Read the model definition and answer for the solid it produces. Units are mm, in the model's axes. A direction names the side the tool comes from. Give positions to 0.01 mm unless a question says otherwise; leave off trailing zeros. Order: outer loops, then holes, each group sorted by start corner. A loop starts at its lowest first (then second) coordinate and runs counter-clockwise, first axis right, second up.
```python
from build123d import *

# Parameters (mm, degrees)
OUTER_CLAMP_COVER_62X54X3_SKETCH_R = 1.7
OUTER_CLAMP_COVER_62X54X3_DEPTH    = 3
TWO_CASE_RETAINING_FEET_START      = -2
TWO_CASE_RETAINING_FEET_DEPTH      = 2


with BuildPart() as part:
    # Outer_clamp_cover_62x54x3_Sketch → Outer_clamp_cover_62x54x3 (new body)
    with BuildSketch(Plane.XY):
        with BuildLine():
            Line((-27, -27), (27, -27))
            ThreePointArc((27, -27), (29.828427125, -25.828427125), (31, -23))
            Line((31, -23), (31, 23))
            ThreePointArc((31, 23), (29.828427125, 25.828427125), (27, 27))
            Line((27, 27), (-27, 27))
            ThreePointArc((-27, 27), (-29.828427125, 25.828427125), (-31, 23))
            Line((-31, 23), (-31, -23))
            ThreePointArc((-31, -23), (-29.828427125, -25.828427125), (-27, -27))
        make_face()
        with Locations((-26, -22)):
            Circle(OUTER_CLAMP_COVER_62X54X3_SKETCH_R, mode=Mode.SUBTRACT)
        with Locations((-26, 22)):
            Circle(OUTER_CLAMP_COVER_62X54X3_SKETCH_R, mode=Mode.SUBTRACT)
        with Locations((26, -22)):
            Circle(OUTER_CLAMP_COVER_62X54X3_SKETCH_R, mode=Mode.SUBTRACT)
        with Locations((26, 22)):
            Circle(OUTER_CLAMP_COVER_62X54X3_SKETCH_R, mode=Mode.SUBTRACT)
        with BuildLine():
            Line((-15.9, -12.2), (15.9, -12.2))
            ThreePointArc((15.9, -12.2), (17.667766953, -11.467766953), (18.4, -9.7))
            Line((18.4, -9.7), (18.4, 9.7))
            ThreePointArc((18.4, 9.7), (17.667766953, 11.467766953), (15.9, 12.2))
            Line((15.9, 12.2), (-15.9, 12.2))
            ThreePointArc((-15.9, 12.2), (-17.667766953, 11.467766953), (-18.4, 9.7))
            Line((-18.4, 9.7), (-18.4, -9.7))
            ThreePointArc((-18.4, -9.7), (-17.667766953, -11.467766953), (-15.9, -12.2))
        make_face(mode=Mode.SUBTRACT)
    extrude(amount=OUTER_CLAMP_COVER_62X54X3_DEPTH)

    # Two_case_retaining_feet_Sketch → Two_case_retaining_feet (add)
    with BuildSketch(Plane.XY.offset(TWO_CASE_RETAINING_FEET_START)):
        with BuildLine():
            Line((-14, -17.5), (14, -17.5))
            ThreePointArc((14, -17.5), (14.707106781, -17.207106781), (15, -16.5))
            Line((15, -16.5), (15, -14.6))
            ThreePointArc((15, -14.6), (14.707106781, -13.892893219), (14, -13.6))
            Line((14, -13.6), (-14, -13.6))
            ThreePointArc((-14, -13.6), (-14.707106781, -13.892893219), (-15, -14.6))
            Line((-15, -14.6), (-15, -16.5))
            ThreePointArc((-15, -16.5), (-14.707106781, -17.207106781), (-14, -17.5))
        make_face()
        with BuildLine():
            Line((-14, 13.6), (14, 13.6))
            ThreePointArc((14, 13.6), (14.707106781, 13.892893219), (15, 14.6))
            Line((15, 14.6), (15, 16.5))
            ThreePointArc((15, 16.5), (14.707106781, 17.207106781), (14, 17.5))
            Line((14, 17.5), (-14, 17.5))
            ThreePointArc((-14, 17.5), (-14.707106781, 17.207106781), (-15, 16.5))
            Line((-15, 16.5), (-15, 14.6))
            ThreePointArc((-15, 14.6), (-14.707106781, 13.892893219), (-14, 13.6))
        make_face()
    extrude(amount=TWO_CASE_RETAINING_FEET_DEPTH)


solid = part.part
```
1) The part is cut by section A-A on y = -7.5. Determine the outline of the cut face in (x, z).
Final values:
outline: (-31, 0) - (-18.4, 0) - (-18.4, 3) - (-31, 3) - close; (18.4, 0) - (31, 0) - (31, 3) - (18.4, 3) - close
2) The part is cut by section C-C on x = -26. Determine the outline of the cut face in (y, z), and give its area (3 significant figures).
Final values:
outline: (-27, 0) - (-23.7, 0) - (-23.7, 3) - (-27, 3) - close; (-20.3, 0) - (20.3, 0) - (20.3, 3) - (-20.3, 3) - close; (23.7, 0) - (27, 0) - (27, 3) - (23.7, 3) - close
area: 142 mm2
3) A tool of negligible diameter and unlimited length cuts with its end or side. For faces 4 (the face through (18.4, 0, 1)), 5 (the face through (31, 0, 1)), 6 (the face through (0, 13.6, -1)), 7 (the face through (0, 17.5, -1)), 8 (the face through (0, -17.5, -1)), from which of +Z, -Z, +X, -X, +Y, -Y can it reach the whole face along a straight path? Write none if from no direction.
Final values:
face 4: +Z, -Z
face 5: +Z, -Z, +X, +Y, -Y
face 6: -Z, +X, -X
face 7: -Z, +X, -X, +Y
face 8: -Z, +X, -X, -Y
4) For a pull along Y with two mould halves and no side action, classify faces 1 (the face through (0, -27, 1)), 2 (the face through (-15, -16, -1)), 3 (the face through (-17.648, 11.487, 1.479)) as released by +Y, released by -Y, zero draft, split by the parting line, or undercut.
Final values:
face 1: released by -Y
face 2: zero draft
face 3: undercut
5) Given pin 1 (0.6 mm diameter, centred on y = 15.5, z = -1, fed in from +X); pin 2 (0.6 mm diameter, centred on y = -15.5, z = -0.5, fed in from -X); pin 3 (2 mm diameter, centred on x = -26, y = 22, fed in from -Z); pin 4 (1.6 mm diameter, centred on x = 0.5, z = -1, fed in from -Y), each flat-ended and moving along its own axis, determine where each tip first touches the part or whether it passes through.
Final values:
pin 1: stops at x = 15
pin 2: stops at x = -15
pin 3: passes through
pin 4: stops at y = -17.5
6) The part is cut by section B-B on x = -8. Determine the outline of the cut face in (y, z), and give its area (3 significant figures).
Final values:
outline: (-27, 0) - (-17.5, 0) - (-17.5, -2) - (-13.6, -2) - (-13.6, 0) - (-12.2, 0) - (-12.2, 3) - (-27, 3) - close; (12.2, 0) - (13.6, 0) - (13.6, -2) - (17.5, -2) - (17.5, 0) - (27, 0) - (27, 3) - (12.2, 3) - close
area: 104 mm2
7) The part is cut by section D-D on z = -1.2. Determine the outline of the cut face in (x, y).
Final values:
outline: (-15, -16.5) arc R1 ccw to (-14, -17.5) - (14, -17.5) arc R1 ccw to (15, -16.5) - (15, -14.6) arc R1 ccw to (14, -13.6) - (-14, -13.6) arc R1 ccw to (-15, -14.6) - close; (-15, 14.6) arc R1 ccw to (-14, 13.6) - (14, 13.6) arc R1 ccw to (15, 14.6) - (15, 16.5) arc R1 ccw to (14, 17.5) - (-14, 17.5) arc R1 ccw to (-15, 16.5) - close
8) Consider L1, parallel to Y at x = 26, z = 1.9; L2, parallel to Y at x = -12, z = -1; L3, parallel to X at y = 6, z = 2.55. Determine where each line is inside the solid, lowest interval first.
Final values:
L1: y = -27 to -23.7, -20.3 to 20.3, 23.7 to 27
L2: y = -17.5 to -13.6, 13.6 to 17.5
L3: x = -31 to -18.4, 18.4 to 31
